Geometry check sheet. Reference: drawing and pictorial views, mm from the part's lowest x, y, z. A direction names the side the tool comes from. Give positions to 0.01 mm unless a question says otherwise; leave off trailing zeros. Order: outer loops, then holes, each group sorted by start corner. A loop starts at its lowest first (then second) coordinate and runs counter-clockwise, first axis right, second up.
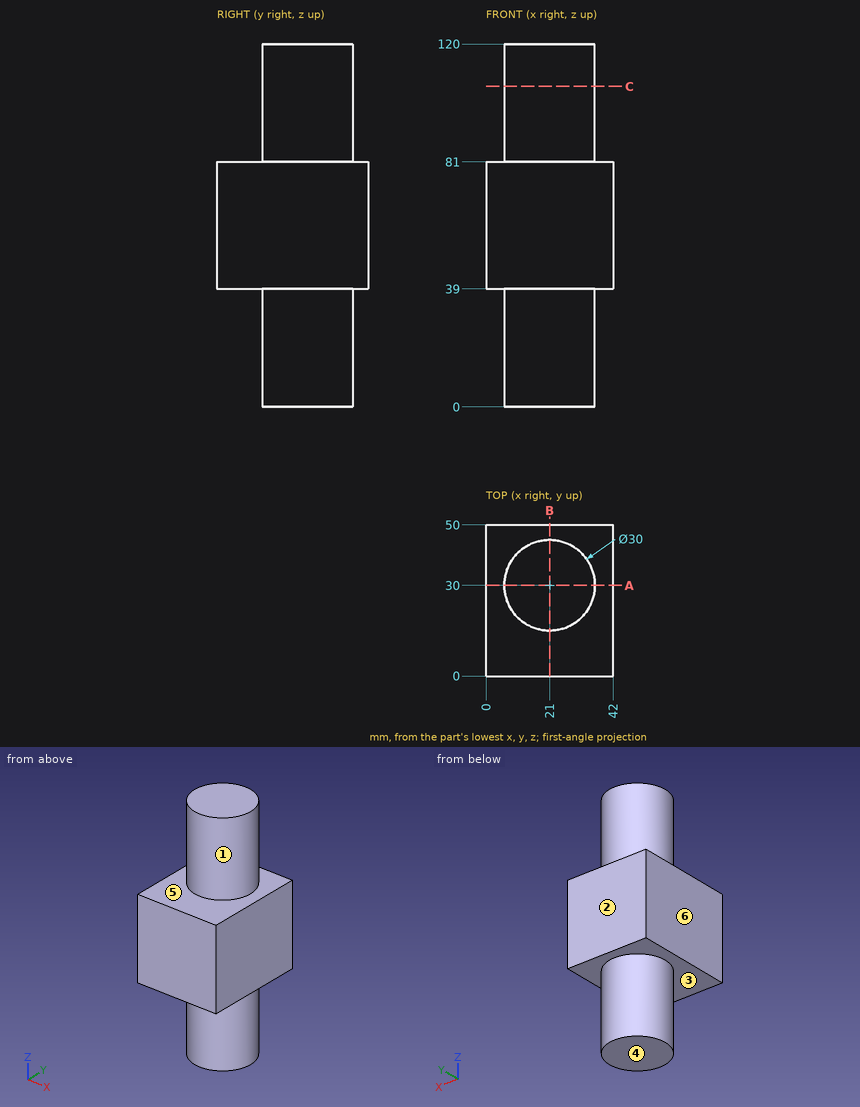
1) Section check B-B, the plane x = 21. Record the cut outline in (y, z), then the cut area to 3 significant figures.
Recorded:
outline: (0, 39) - (15, 39) - (15, 0) - (45, 0) - (45, 39) - (50, 39) - (50, 81) - (45, 81) - (45, 120) - (15, 120) - (15, 81) - (0, 81) - close
area: 4,440 mm2
2) Draft check along Z on the marked faces 4, 5 and 6. Enter one of: +Z half, -Z half, draft (parallel to the pull), parting line (faces both ways), or undercut.
Recorded:
face 4: -Z half
face 5: +Z half
face 6: draft
3) Material ranges on L1, parallel to Z at x = 24.5, y = 11.5; L2, parallel to X at y = 27, z = 27; L3, parallel to Y at x = 24, z = 115, recorded low to high.
Recorded:
L1: z = 39 to 81
L2: x = 6.3 to 35.7
L3: y = 15.3 to 44.7
4) Set-up check for the marked faces 1, 2 and 3: record each of +Z, -Z, +X, -X, +Y, -Y from which the full face is reachable in a straight line by a thin tool's end or side.
Recorded:
face 1: +Z
face 2: +Z, -Z, +X, -X, +Y
face 3: -Z
5) Section check A-A, the plane y = 30. Record the cut outline in (x, z).
Recorded:
outline: (0, 39) - (6, 39) - (6, 0) - (36, 0) - (36, 39) - (42, 39) - (42, 81) - (36, 81) - (36, 120) - (6, 120) - (6, 81) - (0, 81) - close
6) Depth check by flat-ended pin: pin 1 Ø2 at (y, z) = (29.5, 19.5) entering from -X; pin 2 Ø2 at (x, z) = (17.5, 33.5) entering from -Y; pin 3 Ø4 at (y, z) = (44.5, 15) entering from -X. Enter the tip coordinate at first touch or a pass-through.
Recorded:
pin 1: stops at x = 6
pin 2: stops at y = 15.21
pin 3: stops at x = 12.71
7) Section check C-C, the plane z = 106. Record the cut outline in (x, y).
Recorded:
outline: circle Ø30 at (21, 30)
